from build123d import *

# Parameters (mm, degrees)
F0_R     = 27.3478618837
F1_DEPTH = 25.4
F2_W     = 21.4937683195
F2_H     = 14.953751117
F3_DEPTH = 228.6
F4_R     = 65.1026145731
F5_DEPTH = 76.2
F6_R     = 40.595906751
F7_DEPTH = 25.4
F8_R     = 12.7


# Not quite as in the source:
# - a fillet or chamfer that OpenCascade refuses, or shapes differently, is made with other operations: its cross-section is extruded or revolved along the edge and cut away or added


with BuildPart() as f1:
    # F0 (on Top) → F1 (new body)
    with BuildSketch(Plane.XY):
        with Locations((-20.4128082842, 28.926692903)):
            Circle(F0_R)
    extrude(amount=F1_DEPTH)

    # F2 (on face) → F3 (join)
    with BuildSketch(Plane.XY.offset(25.4)):
        with Locations((-20.0721742585, 30.7035986334)):
            Rectangle(F2_W, F2_H)
    extrude(amount=F3_DEPTH)

    # F4 (on face) → F5 (join)
    with BuildSketch(Plane.XZ.offset(-23.2267230749)):
        with Locations((-9.3252900988, 229.8023849726)):
            Circle(F4_R)
    extrude(amount=-F5_DEPTH)

    # F6 (on face) → F7 (cut)
    with BuildSketch(Plane(origin=(0, 99.4267230749, 0), x_dir=(-1, 0, 0), z_dir=(0, 1, 0))):
        with Locations((30.0150513649, 226.0579317808)):
            Circle(F6_R)
    extrude(amount=-F7_DEPTH, mode=Mode.SUBTRACT)

    # F8
    f8_edges = [f1.edges().sort_by_distance(p)[0] for p in [
        (10.580855, 74.026723, 226.057932),
    ]]
    fillet(f8_edges, radius=F8_R)

    # F9: chamfer of 10.16 on 1 edges, made by hand

    # F9_s1 → F9_t2 (revolve, cut)
    with BuildSketch(Plane.XY.offset(229.8023849726)):
        Polygon((45.6173244743, 99.4267230749), (55.7773244743, 89.2667230749), (55.7773244743, 99.4267230749), align=None)
    revolve(axis=Axis((-9.3252900988, 99.4267230749, 229.8023849726), (0, -1, 0)), mode=Mode.SUBTRACT)


solid = f1.part
The listing builds one solid part. Answer for the finished solid, in the listing's coordinates (mm). A direction names the side the tool comes from. Round coordinates to 2 decimals unless told otherwise and drop trailing zeros. Write each loop counter-clockwise with the first axis right and the second up, starting at its lowest first coordinate (ties: lowest second). Pieces come first, ordered by that corner, then holes. Notation, with made-up numbers: (67.5, 71) - (122.5, 71) arc R20 ccw to (122.5, 87) - close; hole circle Ø10 at (46, -10.75). An arc over 180 degrees is marked (long way). Use one line per item in the form item = value. Start each with the question number.
Item 1: A cutting plane is placed at B-B (z = 50). Write down the section's boundary in (x, y), plus the area to 3 significant figures.
Item 2: A cutting plane is placed at D-D (y = 20). Write down the section's boundary in (x, z).
Item 3: A tool of negligible diameter and unlimited length cuts with its end or side. For faces 1 (the cylindrical face through (10.54, 93.17, 227.84)), 2 (the flat face through (-30.819, 31, 96)), 3 (the flat face through (-9.325, 31, 94)), 4 (the flat face through (-10, 23.227, 192)), 5 (the flat face through (-21, 17, 25.4)), from which of +Z, -Z, +X, -X, +Y, -Y can it reach the whole face along a straight path? Write none if from no direction.
Item 4: A cutting plane is placed at C-C (y = 80). Write down the section's boundary in (x, z), plus the area to 3 significant figures.
Item 5: Flat-ended cylindrical pins translate along their axes: pin 1 Ø16.5 at (y, z) = (33, 114.5) entering from -X; pin 2 Ø23.5 at (x, z) = (-22, 94) entering from +Y; pin 3 Ø4 at (x, y) = (-39.5, 52) entering from +Z. Find the tip coordinate at first contact, or state that the pin passes through.
Item 6: Find the intervals of material crossed by line 1 (Y direction, x = -38.5, z = 200); line 2 (X direction, y = 81, z = 245.5); line 3 (Y direction, x = -27.5, z = 96), in increasing order. Write a range as [from, to].
Item 7: A cutting plane is placed at A-A (y = 44.5). Write down the section's boundary in (x, z), plus the area to 3 significant figures.
The answers:
q1.outline = (-30.82, 23.23) - (-9.33, 23.23) - (-9.33, 38.18) - (-30.82, 38.18) - close
q1.area = 321 mm^2
q2.outline = (-46.26, 0) - (5.44, 0) - (5.44, 25.4) - (-46.26, 25.4) - close
q3.face_1 = +Y
q3.face_2 = -X, +Y, -Y
q3.face_3 = +X, +Y, -Y
q3.face_4 = +Z, +X, -X, -Y
q3.face_5 = none
q4.outline = circle Ø130.21 at (-9.33, 229.8); hole circle Ø77.34 at (-30.02, 226.06)
q4.area = 8,620 mm^2
q5.pin_1 = -30.82
q5.pin_2 = 38.18
q5.pin_3 = 288.49
q6.line_1 = [23.23, 74.03]
q6.line_2 = [-72.51, -64.09], [4.06, 53.86]
q6.line_3 = [23.23, 38.18]
q7.outline = circle Ø130.21 at (-9.33, 229.8); (-42.89, 0) - (2.07, 0) - (2.07, 25.4) - (-42.89, 25.4) - close
q7.area = 14,500 mm^2
